Work out the finished part from the listing and answer in its coordinate system (mm). Face numbers are marked on the shaded views. A direction names the side the tool comes from. Give positions to 0.01 mm unless a question says otherwise; leave off trailing zeros. Loops run counter-clockwise (first coordinate to the right, second up) from the corner with the lowest first, then second, coordinate; pieces in that order, holes last. Notation, with made-up numbers: (2, -8.5) - (7, -8.5) arc R6 cw to (7, -4.5) - close; hole circle Ø9 at (19.5, 72.25). An arc over 180 degrees is marked (long way). One line per question, with ' | ' between items. Start each with the question number.
1. Section A-A (y = 34.5) is taken. Determine the outline of the cut face in (x, z), plus the area to 3 significant figures.
2. Each of these flat-tipped pins is pushed along its axis until it touches: pin 1 (3 mm diameter, centred on y = 10.5, z = -7, fed in from +X); pin 2 (15 mm diameter, centred on x = 11, y = 5, fed in from +Z); pin 3 (2.5 mm diameter, centred on x = 18.5, z = 18, fed in from +Y). Where does it stop, or does it pass through?
3. For a pull along X with two mould halves and no side action, classify the marked faces 1, 2 and 3 as released by +X, released by -X, zero draft, split by the parting line, or undercut.
4. Section C-C (z = 22) is taken. Determine the outline of the cut face in (x, y), plus the area to 3 significant figures.
5. Which of the six approach directions +Z, -Z, +X, -X, +Y, -Y give full straight-line access (tool end or side, diameter ignored) to the marked faces 4, 5 and 6?
6. Section D-D (y = 7) is taken. Determine the outline of the cut face in (x, z), plus the area to 3 significant figures.
7. Find the intervals of material crossed by line 1 (Z direction, x = 32, y = 35); line 2 (Z direction, x = 31.75, y = 32.75); line 3 (Z direction, x = 35.5, y = 8), in increasing order.
8. Section B-B (x = 16.5) is taken. Determine the outline of the cut face in (y, z).
Autodesk Inventor part; units mm, degrees
ref_plane "YZ Plane" through (0, 0, 0) normal (1, 0, 0) x (0, 1, 0)
ref_plane "XZ Plane" through (0, 0, 0) normal (0, 1, 0) x (-1, 0, 0)
ref_plane "XY Plane" through (0, 0, 0) normal (0, 0, 1) x (1, 0, 0)
sketch "Sketch1" plane through (0, 0, 0) normal (0, 0, 1) x (1, 0, 0)
  line L0 (0, 0) -> (38.1, 0)
  line L1 (38.1, 0) -> (38.1, 38.1)
  line L2 (38.1, 38.1) -> (0, 38.1)
  line L3 (0, 38.1) -> (0, 0)
  circle A0 centre (19.05, 19.05) radius 6.35
  line L4 (20.6375, 23.8125) -> (17.4625, 23.8125)
  line L5 (17.4625, 25.4) -> (20.6375, 25.4)
  line L6 (20.6375, 23.8125) -> (20.6375, 25.4)
  line L7 (17.4625, 23.8125) -> (17.4625, 25.4)
  circle A1 centre (19.05, 19.05) radius 19.05
  point P0 (19.05, 0)
  point P1 (0, 19.05)
  point P2 (19.05, 23.8125)
  dimension "d0" = 38.1
  dimension "d1" = 38.1
  dimension "d2" = 12.7
  dimension "d3" = 3.175
extrude "Extrusion1" add sketch "Sketch1" along normal blind 12.7 contours L3 A1 L0 | A1 L1 L0 | A1 | L3 L2 A1 | A1 L2 L1 | A0 L7 L4 L6 | L6 L4 L7 A0
extrude "Extrusion2" add sketch "Sketch1" along normal blind 50.8 contours A0 L7 L4 L6 | L6 L4 L7 A0
extrude "Extrusion3" cut sketch "Sketch1" along normal blind 50.8 contours L6 L4 L7 A0 | A0 L5 L6 | L7 L5 A0 picked at (19.05, 24.3417)
extrude "Extrusion4" add sketch "Sketch1" against normal blind 38.1 contours A1
sketch "Sketch2" plane through (19.05, 19.05, -38.1) normal (0, 0, -1) x (-1, 0, 0)
  arc A0 (-1.5875, 6.1484) -> (1.5875, 6.1484) centre (0, 0) ccw
  line L0 (-1.5875, 6.1484) -> (-1.5875, 6.35)
  line L1 (-1.5875, 6.35) -> (1.5875, 6.35)
  line L2 (1.5875, 6.35) -> (1.5875, 6.1484)
  circle A1 centre (0, 0) radius 19.05
  line L3 (-19.05, 19.05) -> (19.05, 19.05)
  line L4 (19.05, 19.05) -> (19.05, -19.05)
  line L5 (19.05, -19.05) -> (-19.05, -19.05)
  line L6 (-19.05, -19.05) -> (-19.05, 19.05)
extrude "Extrusion5" add sketch "Sketch2" along normal blind 13.97
sketch "Sketch3" plane through (0, 38.1, 12.7) normal (0, 1, 0) x (1, 0, 0)
  line L0 (0, 0) -> (38.1, 0)
  line L1 (0, 12.7) -> (0, 0)
  point P0 (31.75, 6.35)
  point P1 (6.35, 6.35)
  point P2 (6.35, 58.42)
  point P3 (31.75, 58.42)
  point P4 (0, 64.77)
  dimension "d15" = 6.35
  dimension "d16" = 25.4
  dimension "d17" = 6.35
  dimension "d18" = 6.35
hole "Hole1" at (31.75, 38.1, 6.35) at (6.35, 38.1, 6.35) at (6.35, 38.1, -45.72) at (31.75, 38.1, -45.72) direction (0, -1, 0) diameter 4.7625 depth 12.7 tip angle 118
thread "Thread1"
thread "Thread2"
thread "Thread3"
thread "Thread4"
properties part number "hack_p60"
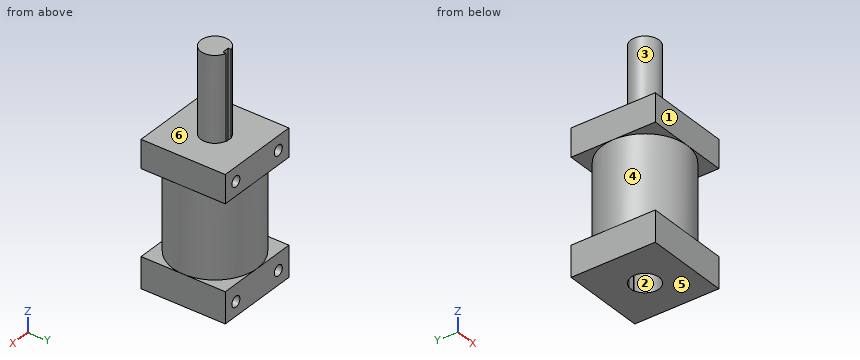
Conclusion:
1) outline: (0, -52.07) - (38.1, -52.07) - (38.1, -38.1) - (30.19, -38.1) - (30.19, 0) - (38.1, 0) - (38.1, 12.7) - (0, 12.7) - (0, 0) - (7.91, 0) - (7.91, -38.1) - (0, -38.1) - close; hole circle Ø4.76 at (6.35, -45.72); hole circle Ø4.76 at (6.35, 6.35); hole circle Ø4.76 at (31.75, -45.72); hole circle Ø4.76 at (31.75, 6.35) | area: 1,790 mm²
2) pin 1: x = 36.75 | pin 2: z = 12.7 | pin 3: y = 25.2
3) face 1: zero draft | face 2: undercut | face 3: split by the parting line
4) outline: (17.46, 23.81) - (17.46, 25.2) arc R6.35 ccw (long way) to (20.64, 25.2) - (20.64, 23.81) - close | area: 122 mm²
5) face 4: none | face 5: -Z, +X, -X, +Y, -Y | face 6: +Z
6) outline: (0, -52.07) - (38.1, -52.07) - (38.1, -38.1) - (33.8, -38.1) - (33.8, 0) - (38.1, 0) - (38.1, 12.7) - (0, 12.7) - (0, 0) - (4.3, 0) - (4.3, -38.1) - (0, -38.1) - close | area: 2,140 mm²
7) line 1: -52.07 to -48.09, -43.35 to -38.1, 0 to 3.98, 8.72 to 12.7 | line 2: -52.07 to -48.1, -43.34 to 3.97, 8.73 to 12.7 | line 3: -52.07 to -38.1, 0 to 12.7
8) outline: (0, -52.07) - (13.23, -52.07) - (13.23, 0) - (24.87, 0) - (24.87, -52.07) - (38.1, -52.07) - (38.1, -38.1) - (37.93, -38.1) - (37.93, 0) - (38.1, 0) - (38.1, 12.7) - (24.87, 12.7) - (24.87, 50.8) - (13.23, 50.8) - (13.23, 12.7) - (0, 12.7) - (0, 0) - (0.17, 0) - (0.17, -38.1) - (0, -38.1) - close
